Design review of the part shown in the three views and the two pictorial views. Dimensions are in mm from the part's minimum x, y and z. A direction names the side the tool comes from. Coordinates: 2 decimals unless noted, no trailing zeros. Write each loop counter-clockwise with the first axis right and the second up, starting at its lowest first coordinate (ties: lowest second). Pieces come first, ordered by that corner, then holes.
Q1. Take a section at A-A, the plane x = 69. Write out the cut boundary in (y, z) (3 decimals), plus the area to 3 significant figures.
Q2. The part is to be moulded in two halves that separate along X. For the marked faces 1, 2 and 3, say which applies: released by +X, released by -X, zero draft, split by the parting line, or undercut.
Q3. For the marked faces 4, 5 and 6, list the 3-axis set-ups (+Z, -Z, +X, -X, +Y, -Y) from which the entire face can be reached by the end or side of a thin tool; tool diameter is ignored.
Q4. For L1, parallel to Y at x = 19, z = 9; L2, parallel to Z at x = 31, y = 5; L3, parallel to Z at x = 57.5, y = 22, list the stretches that pass through material, from the lowest coordinate up.
Q5. Take a section at D-D, the plane x = 19.05. Write out the cut boundary in (y, z), plus the area to 3 significant figures.
Q6. For pin 1 Ø12 at (x, y) = (15.5, 26.5) entering from +Z; pin 2 Ø16 at (x, y) = (79, 23) entering from -Z; pin 3 Ø4 at (y, z) = (23.5, 9.5) entering from +X, all flat-tipped, find the tip position at first contact; note any pin that passes through.
Q7. Take a section at B-B, the plane y = 28.5. Write out the cut boundary in (x, z).
Q8. Take a section at C-C, the plane y = 20.5. Write out the cut boundary in (x, z).
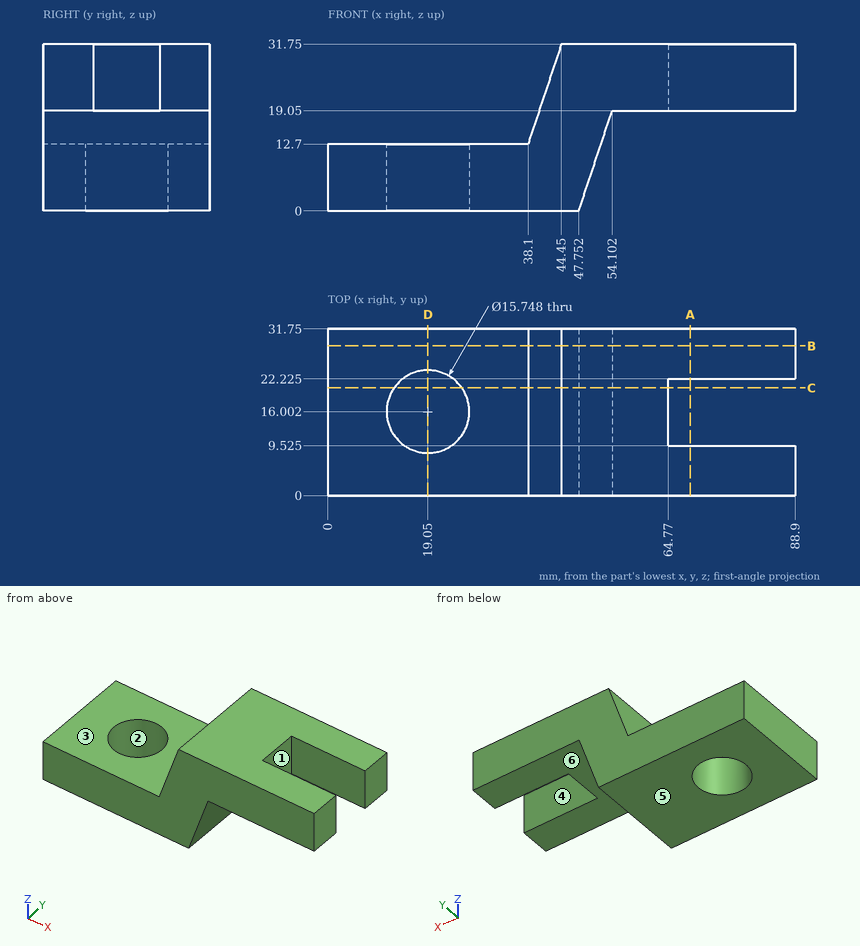
Responses:
1. outline: (0, 19.05) - (9.525, 19.05) - (9.525, 31.75) - (0, 31.75) - close; (22.225, 19.05) - (31.75, 19.05) - (31.75, 31.75) - (22.225, 31.75) - close
1. area: 242 mm2
2. face 1: released by +X
2. face 2: undercut
2. face 3: zero draft
3. face 4: +Z, -Z, +X
3. face 5: -Z, +X, -X, +Y, -Y
3. face 6: -Z, +X, +Y, -Y
4. L1: y = 0 to 8.13, 23.88 to 31.75
4. L2: z = 0 to 12.7
4. L3: z = 19.05 to 31.75
5. outline: (0, 0) - (8.13, 0) - (8.13, 12.7) - (0, 12.7) - close; (23.88, 0) - (31.75, 0) - (31.75, 12.7) - (23.88, 12.7) - close
5. area: 203 mm2
6. pin 1: stops at z = 12.7
6. pin 2: stops at z = 19.05
6. pin 3: stops at x = 51.59
7. outline: (0, 0) - (47.75, 0) - (54.1, 19.05) - (88.9, 19.05) - (88.9, 31.75) - (44.45, 31.75) - (38.1, 12.7) - (0, 12.7) - close
8. outline: (0, 0) - (12.59, 0) - (12.59, 12.7) - (0, 12.7) - close; (25.51, 0) - (47.75, 0) - (54.1, 19.05) - (64.77, 19.05) - (64.77, 31.75) - (44.45, 31.75) - (38.1, 12.7) - (25.51, 12.7) - close
